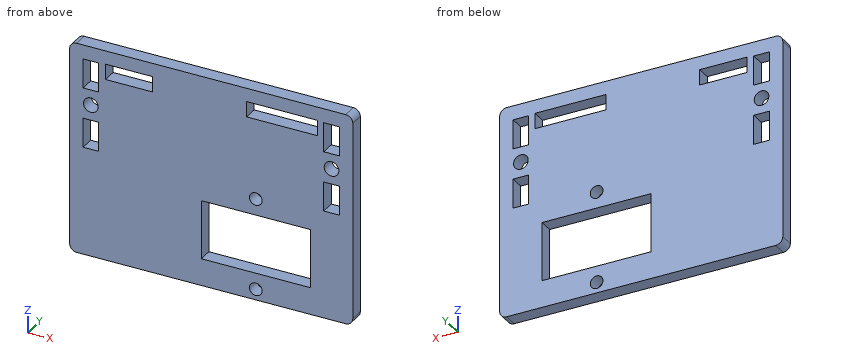
from build123d import *

# Parameters (mm, degrees)
BOSS_EXTRUDE1_DEPTH     = 3
SKETCH2_R               = 1.35
SKETCH2_R_2             = 1.55
SKETCH2_W               = 23.1
SKETCH2_H               = 12.5
SKETCH2_W_2             = 15
SKETCH2_H_2             = 3
SKETCH2_W_3             = 10
SKETCH2_W_4             = 3
SKETCH2_H_3             = 6.25
MAIN_HOLE_EXTRUDE_DEPTH = 4
SKETCH3_W               = 10
SKETCH3_H               = 0.15
SKETCH3_W_2             = 15
SKETCH3_W_3             = 0.15
SKETCH3_H_2             = 6.25
CLEARANCE_EXTRUDE_DEPTH = 4


with BuildPart() as part:
    # Sketch1 → Boss-Extrude1 (new body)
    with BuildSketch(Plane(origin=(0, 0, 0), x_dir=(1, 0, 0), z_dir=(0, 1, 0))):
        with BuildLine():
            Line((1.5, 0), (58.5, 0))
            ThreePointArc((58.5, 0), (59.560660172, 0.439339828), (60, 1.5))
            Line((60, 1.5), (60, 43.5))
            ThreePointArc((60, 43.5), (59.560660172, 44.560660172), (58.5, 45))
            Line((58.5, 45), (1.5, 45))
            ThreePointArc((1.5, 45), (0.439339828, 44.560660172), (0, 43.5))
            Line((0, 43.5), (0, 1.5))
            ThreePointArc((0, 1.5), (0.439339828, 0.439339828), (1.5, 0))
        make_face()
    extrude(amount=BOSS_EXTRUDE1_DEPTH)

    # Sketch2 → Main Hole Extrude (cut, through all)
    with BuildSketch(Plane(origin=(0, 3, 0), x_dir=(1, 0, 0), z_dir=(0, 1, 0))):
        with Locations((39.45, 23.3)):
            Circle(SKETCH2_R)
        with Locations((39.45, 42.7)):
            Circle(SKETCH2_R)
        with Locations((4.5, 12.5)):
            Circle(SKETCH2_R_2)
        with Locations((55.5, 12.5)):
            Circle(SKETCH2_R_2)
        with Locations((39.45, 33)):
            Rectangle(SKETCH2_W, SKETCH2_H)
        with Locations((45, 4.5)):
            Rectangle(SKETCH2_W_2, SKETCH2_H_2)
        with Locations((12.6, 4.5)):
            Rectangle(SKETCH2_W_3, SKETCH2_H_2)
        with Locations((4.5, 18.875)):
            Rectangle(SKETCH2_W_4, SKETCH2_H_3)
        with Locations((4.5, 6.125)):
            Rectangle(SKETCH2_W_4, SKETCH2_H_3)
        with Locations((55.5, 18.875)):
            Rectangle(SKETCH2_W_4, SKETCH2_H_3)
        with Locations((55.5, 6.125)):
            Rectangle(SKETCH2_W_4, SKETCH2_H_3)
    extrude(amount=-MAIN_HOLE_EXTRUDE_DEPTH, mode=Mode.SUBTRACT)

    # Sketch3 → Clearance Extrude (cut, through all)
    with BuildSketch(Plane(origin=(0, 3, 0), x_dir=(1, 0, 0), z_dir=(0, 1, 0))):
        with Locations((12.6, 6.075)):
            Rectangle(SKETCH3_W, SKETCH3_H)
        with Locations((12.6, 2.925)):
            Rectangle(SKETCH3_W, SKETCH3_H)
        with Locations((45, 6.075)):
            Rectangle(SKETCH3_W_2, SKETCH3_H)
        with Locations((45, 2.925)):
            Rectangle(SKETCH3_W_2, SKETCH3_H)
        with Locations((6.075, 18.875)):
            Rectangle(SKETCH3_W_3, SKETCH3_H_2)
        with Locations((2.925, 18.875)):
            Rectangle(SKETCH3_W_3, SKETCH3_H_2)
        with Locations((6.075, 6.125)):
            Rectangle(SKETCH3_W_3, SKETCH3_H_2)
        with Locations((2.925, 6.125)):
            Rectangle(SKETCH3_W_3, SKETCH3_H_2)
        with Locations((53.925, 18.875)):
            Rectangle(SKETCH3_W_3, SKETCH3_H_2)
        with Locations((57.075, 18.875)):
            Rectangle(SKETCH3_W_3, SKETCH3_H_2)
        with Locations((57.075, 6.125)):
            Rectangle(SKETCH3_W_3, SKETCH3_H_2)
        with Locations((53.925, 6.125)):
            Rectangle(SKETCH3_W_3, SKETCH3_H_2)
    extrude(amount=-CLEARANCE_EXTRUDE_DEPTH, mode=Mode.SUBTRACT)


solid = part.part
Read the model definition and answer for the solid it produces. Units are mm, in the model's axes. Coordinates: 2 decimals unless noted, no trailing zeros. Order: outer loops, then holes, each group sorted by start corner. A loop starts at its lowest first (then second) coordinate and runs counter-clockwise, first axis right, second up. Notation, with made-up numbers: (10.5, -38) - (57.5, -38) arc R5 ccw to (57.5, -29) - close; hole circle Ø6 at (57, -5). An arc over 180 degrees is marked (long way). Use one line per item in the form item = value.
(1) Section B-B, the plane z = -12.5 is taken. Give the vertices of the cut face in (x, y), then the cut area to 3 significant figures.
Computed values:
outline = (0, 0) - (2.95, 0) - (2.95, 3) - (0, 3) - close; (6.05, 0) - (53.95, 0) - (53.95, 3) - (6.05, 3) - close; (57.05, 0) - (60, 0) - (60, 3) - (57.05, 3) - close
area = 161 mm²
(2) Section A-A, the plane x = 39.45 is taken. Give the vertices of the cut face in (y, z).
Computed values:
outline = (0, -45) - (3, -45) - (3, -44.05) - (0, -44.05) - close; (0, -41.35) - (3, -41.35) - (3, -39.25) - (0, -39.25) - close; (0, -26.75) - (3, -26.75) - (3, -24.65) - (0, -24.65) - close; (0, -21.95) - (3, -21.95) - (3, -6.15) - (0, -6.15) - close; (0, -2.85) - (3, -2.85) - (3, 0) - (0, 0) - close
(3) Given pin 1 Ø1.5 at (x, z) = (38, -24) entering from -Y, flat-ended and moving along its own axis, determine where the tip first touches the part or whether it passes through.
Computed values:
pin_1 = 0
(4) Straight lines are drawn through the part: L1, parallel to X at y = 2.3, z = -12.5; L2, parallel to X at y = 1.05, z = -8.5; L3, parallel to Z at x = 44, y = 1.9. For each, find the intervals that lie inside material, in ascending order.
Computed values:
L1 = 0 to 2.95, 6.05 to 53.95, 57.05 to 60
L2 = 0 to 2.85, 6.15 to 53.85, 57.15 to 60
L3 = -45 to -39.25, -26.75 to -6.15, -2.85 to 0
(5) Section C-C, the plane x = 4.5 is taken. Give the vertices of the cut face in (y, z).
Computed values:
outline = (0, -45) - (3, -45) - (3, -22) - (0, -22) - close; (0, -15.75) - (3, -15.75) - (3, -14.05) - (0, -14.05) - close; (0, -10.95) - (3, -10.95) - (3, -9.25) - (0, -9.25) - close; (0, -3) - (3, -3) - (3, 0) - (0, 0) - close
(6) Section D-D, the plane z = -23.3 is taken. Give the vertices of the cut face in (x, y), then the cut area to 3 significant figures.
Computed values:
outline = (0, 0) - (38.1, 0) - (38.1, 3) - (0, 3) - close; (40.8, 0) - (60, 0) - (60, 3) - (40.8, 3) - close
area = 172 mm²
